Can you work these out from the model? Positions are in its coordinate system, mm. Face numbers are marked on the shaded views. A direction names the side the tool comes from. Give positions to 0.01 mm unless a question says otherwise; leave off trailing zeros. Order: outer loops, then holes, each group sorted by start corner. A loop starts at its lowest first (then second) coordinate and runs counter-clockwise, first axis right, second up. Notation, with made-up numbers: (61.5, 44.25) - (88.5, 44.25) arc R21 cw to (88.5, 83.25) - close; hole circle Ø9 at (20.5, -17). An arc over 180 degrees is marked (long way). One line per question, with ' | ' between items.
```python
from build123d import *

# Parameters (mm, degrees)
SKETCH1_W           = 3.9116
SKETCH1_H           = 4.7752
SKETCH2_R           = 2.3876
BOSS_EXTRUDE1_DEPTH = 12.7
CUT_EXTRUDE1_DEPTH  = 2.794
CHAMFER1_SIZE       = 0.508
CHAMFER2_SIZE       = 0.254


with BuildPart() as part:
    # Sketch1 → Revolve1 (revolve)
    with BuildSketch(Plane.XY, mode=Mode.PRIVATE) as revolve1_sk:
        with Locations((-1.9558, -2.3876)):
            Rectangle(SKETCH1_W, SKETCH1_H)
    revolve(revolve1_sk.sketch.rotate(Axis((0, -4.7752, 0), (0, 1, 0)), 90), axis=Axis((0, -4.7752, 0), (0, 1, 0)))

    # Sketch2 → Boss-Extrude1 (add)
    with BuildSketch(Plane.XZ.offset(4.7752)):
        with Locations(Location((0, 0, 0), (0, 0, 270))):
            Circle(SKETCH2_R)
    extrude(amount=BOSS_EXTRUDE1_DEPTH)

    # Sketch3 → Cut-Extrude1 (cut)
    with BuildSketch(Plane(origin=(0, 0, 0), x_dir=(-1, 0, 0), z_dir=(0, 1, 0))):
        Polygon((1.984374999, -1.14567944), (1.984374999, 1.14567944), (0, 2.29135888), (-1.984374999, 1.14567944), (-1.984374999, -1.14567944), (0, -2.29135888), align=None)
    extrude(amount=-CUT_EXTRUDE1_DEPTH, mode=Mode.SUBTRACT)

    # Chamfer1
    chamfer1_edges = [part.edges().sort_by_distance(p)[0] for p in [
        (0, 0, -3.9116),
        (0, -17.4752, 2.3876),
    ]]
    chamfer(chamfer1_edges, length=CHAMFER1_SIZE)

    # Chamfer2
    chamfer2_edges = [part.edges().sort_by_distance(p)[0] for p in [
        (-0.9921875, 0, -1.71851916),
        (-1.984374999, 0, 0),
        (-0.9921875, 0, 1.71851916),
        (0.9921875, 0, 1.71851916),
        (1.984374999, 0, 0),
        (0.9921875, 0, -1.71851916),
    ]]
    chamfer(chamfer2_edges, length=CHAMFER2_SIZE)


solid = part.part
```
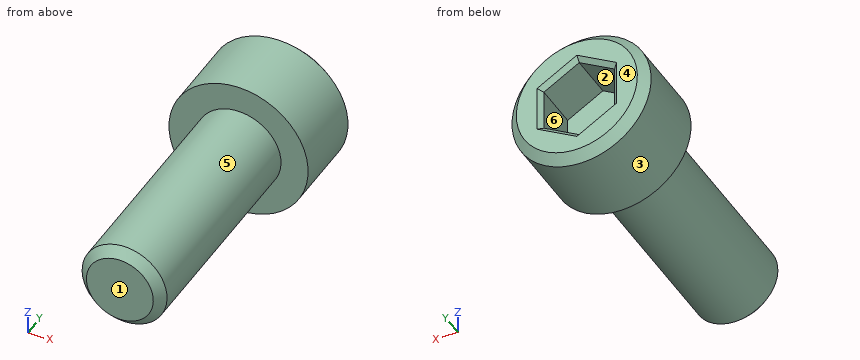
(1) On a 3-axis mill with a long thin cutter (end or side, diameter ignored), from which of +Z, -Z, +X, -X, +Y, -Y can I reach the whole of each face in a straight line? I mean the marked faces 4, 5 and 6. Say none if no direction works.
Answer below:
face 4: +Z, -Z, +X, -X, +Y | face 5: -Y | face 6: +Y
(2) If I drill on line 1 (Y direction, x = -1.25, z = 2.25); line 2 (X direction, y = -10, z = 0); line 3 (Z direction, x = -1.75, y = -5.5), over which ranges is the centre line in solid material (lowest first)?
Answer below:
line 1: -4.78 to 0 | line 2: -2.39 to 2.39 | line 3: -1.62 to 1.62
(3) Imagine slicing it at C-C (y = -8). List the corners of the cut face in (x, z) for me, and give its area (3 significant figures).
Answer below:
outline: circle Ø4.78 at (0, 0) | area: 17.9 mm^2
(4) Imagine slicing it at A-A (y = -2.5). List the corners of the cut face in (x, z) for me, and give its area (3 significant figures).
Answer below:
outline: circle Ø7.82 at (0, 0); hole (-1.98, -1.15) - (0, -2.29) - (1.98, -1.15) - (1.98, 1.15) - (0, 2.29) - (-1.98, 1.15) - close | area: 34.4 mm^2
(5) Will these pins go through, and if not, where does the flat tip stop? pin 1 (2 mm diameter, centred on x = 3, y = -7.5, fed in from -Z); pin 2 (1.5 mm diameter, centred on x = 1.5, y = -6.5, fed in from -Z); pin 3 (4 mm diameter, centred on y = -9.5, z = 1, fed in from -X).
Answer below:
pin 1: z = -1.3 | pin 2: z = -2.27 | pin 3: x = -2.39
(6) If we mould it in two halves opening along X, with no side actions, what happens to the marked faces 1, 2 and 3? For each: released by +X, released by -X, zero draft, split by the parting line, or undercut.
Answer below:
face 1: zero draft | face 2: undercut | face 3: split by the parting line
(7) Imagine slicing it at B-B (z = 0). List the corners of the cut face in (x, y) for me, and give its area (3 significant figures).
Answer below:
outline: (-3.91, -4.78) - (-2.39, -4.78) - (-2.39, -16.97) - (-1.88, -17.48) - (1.88, -17.48) - (2.39, -16.97) - (2.39, -4.78) - (3.91, -4.78) - (3.91, -0.51) - (3.4, 0) - (2.24, 0) - (1.98, -0.25) - (1.98, -2.79) - (-1.98, -2.79) - (-1.98, -0.25) - (-2.24, 0) - (-3.4, 0) - (-3.91, -0.51) - close | area: 86.3 mm^2
